Geometry check sheet. Reference: the model listing, model coordinates, mm. Face numbers are marked on the shaded views. A direction names the side the tool comes from. Round coordinates to 2 decimals unless told otherwise and drop trailing zeros. Write each loop counter-clockwise with the first axis right and the second up, starting at its lowest first coordinate (ties: lowest second). Pieces come first, ordered by that corner, then holes.
Item 1: Cross-section at D-D (z = 15). Enter the section's corners in (x, y) (3 decimals).
Item 2: Draft check along Z on the marked faces 1, 2 and 3. Enter one of: pulls with the +Z half, pulls with the -Z half, needs draft (parallel to the pull), parting line crosses it, or undercut.
Item 3: Scan lines: probe 1 along Y at (x, z) = (-0.2, -6.5); probe 2 along X at (y, z) = (5.75, 9) (3 decimals); probe 3 along Y at (x, z) = (-3, 14). Record each from-to range of solid material in increasing order.
Item 4: Access from +Z, -Z, +X, -X, +Y, -Y to the whole of each face (thin tool, end or side, straight path). Record for the marked faces 4, 5, 6, 7 and 8.
Item 5: Cross-section at C-C (y = 5.5). State how many separate pieces and enclosed holes the cut face has, then the cut area to 3 significant figures.
Item 6: Depth check by flat-ended pin: P1, Ø10, axis at x = -5.5, y = 4, coming from the -Z side; P2, Ø7, axis at y = 5, z = -6.5, coming from the +X side; P3, Ø3, axis at y = 6.5, z = -2.5, coming from the -X side; P4, Ø5, axis at y = 5.5, z = -2, coming from the +X side. Enter the tip coordinate at first touch or a pass-through.
Item 7: Cross-section at B-B (z = 10). Enter the section's corners in (x, y) (3 decimals), then the cut area to 3 significant figures.
Item 8: Cross-section at A-A (z = -4). Enter the section's corners in (x, y).
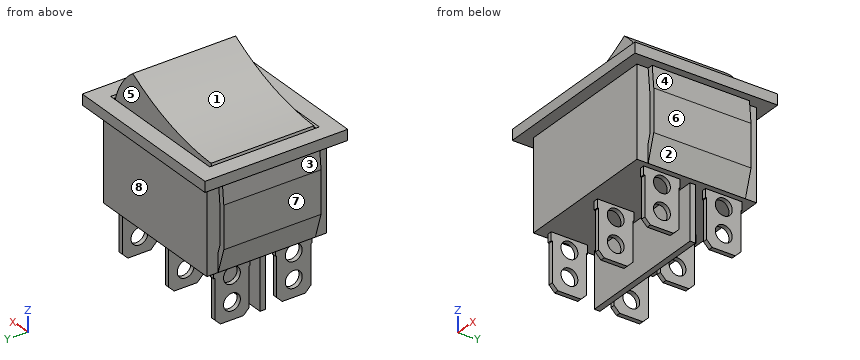
from build123d import *

# Parameters (mm, degrees)
SKETCH1_W                = 25.75
SKETCH1_H                = 21.3
BOSS_EXTRUDE1_DEPTH      = 16
SKETCH3_W                = 30.5
SKETCH3_H                = 25.4
BOSS_EXTRUDE3_DEPTH      = 1.87
SKETCH4_W                = 23.8
SKETCH4_H                = 1
BOSS_EXTRUDE4_DEPTH      = 9.8
SKETCH5_W                = 0.8
SKETCH5_H                = 6.5
BOSS_EXTRUDE5_DEPTH      = 9.5
SKETCH6_W                = 8
SKETCH6_H                = 0.2
CUT_EXTRUDE1_DEPTH       = 35.896266276
CHAMFER1_SIZE            = 1
SKETCH7_R                = 1.5
CUT_EXTRUDE2_DEPTH       = 35.896266276
CHAMFER1_OF_MIRROR1_SIZE = 1
BOSS_EXTRUDE6_START      = -2
BOSS_EXTRUDE6_DEPTH      = 17.3
SKETCH9_W                = 24
SKETCH9_H                = 18.9
CUT_EXTRUDE3_DEPTH       = 5
SKETCH10_R               = 12.5
BOSS_EXTRUDE7_DEPTH      = 9.15
CUT_EXTRUDE4_DEPTH       = 34.003475575
CUT_EXTRUDE4_DEPTH_BACK  = 34.003475575
SKETCH11_R               = 40
CHAMFER2_SIZE            = 0.3


with BuildPart() as part:
    # Sketch1 → Boss-Extrude1 (new body)
    with BuildSketch(Plane.XY):
        Rectangle(SKETCH1_W, SKETCH1_H)
    extrude(amount=BOSS_EXTRUDE1_DEPTH)

    # Sketch3 → Boss-Extrude3 (add)
    with BuildSketch(Plane.XY.offset(16)):
        Rectangle(SKETCH3_W, SKETCH3_H)
    extrude(amount=BOSS_EXTRUDE3_DEPTH)

    # Sketch4 → Boss-Extrude4 (add)
    with BuildSketch(Plane(origin=(0, 0, 0), x_dir=(-1, 0, 0), z_dir=(0, 0, -1))):
        Rectangle(SKETCH4_W, SKETCH4_H)
    extrude(amount=BOSS_EXTRUDE4_DEPTH)

    # Sketch5 → Boss-Extrude5 (add)
    with BuildSketch(Plane(origin=(0, 0, 0), x_dir=(-1, 0, 0), z_dir=(0, 0, -1))):
        with Locations((11.5, -5.5)):
            Rectangle(SKETCH5_W, SKETCH5_H)
        with Locations((0, -5.5)):
            Rectangle(SKETCH5_W, SKETCH5_H)
        with Locations((-11.5, -5.5)):
            Rectangle(SKETCH5_W, SKETCH5_H)
    boss_extrude5 = extrude(amount=BOSS_EXTRUDE5_DEPTH)

    # Sketch6 → Cut-Extrude1 (cut, through all)
    with BuildSketch(Plane(origin=(11.9, 0, 0), x_dir=(0, 0, -1), z_dir=(1, 0, 0))):
        with Locations((5.5, -2.35)):
            Rectangle(SKETCH6_W, SKETCH6_H)
        with Locations((5.5, -8.65)):
            Rectangle(SKETCH6_W, SKETCH6_H)
    cut_extrude1 = extrude(amount=-CUT_EXTRUDE1_DEPTH, mode=Mode.SUBTRACT)

    # Chamfer1
    chamfer1_edges = [part.edges().sort_by_distance(p)[0] for p in [
        (-11.5, -2.45, -9.5),
        (0, -2.45, -9.5),
        (-11.5, -8.55, -9.5),
        (0, -8.55, -9.5),
        (11.5, -8.55, -9.5),
        (11.5, -2.45, -9.5),
    ]]
    chamfer(chamfer1_edges, length=CHAMFER1_SIZE)

    # Sketch7 → Cut-Extrude2 (cut, through all)
    with BuildSketch(Plane(origin=(11.9, 0, 0), x_dir=(0, 0, -1), z_dir=(1, 0, 0))):
        with Locations((6.5, -5.5)):
            Circle(SKETCH7_R)
        with Locations((2, -5.5)):
            Circle(SKETCH7_R)
    cut_extrude2 = extrude(amount=-CUT_EXTRUDE2_DEPTH, mode=Mode.SUBTRACT)

    # Mirror1: Boss-Extrude5, Cut-Extrude1, Cut-Extrude2 across plane
    add(boss_extrude5.mirror(Plane(origin=(0, 0, 0), x_dir=(0, 0, 1), z_dir=(0, -1, 0))))
    add(cut_extrude1.mirror(Plane(origin=(0, 0, 0), x_dir=(0, 0, 1), z_dir=(0, -1, 0))), mode=Mode.SUBTRACT)
    add(cut_extrude2.mirror(Plane(origin=(0, 0, 0), x_dir=(0, 0, 1), z_dir=(0, -1, 0))), mode=Mode.SUBTRACT)

    # Chamfer1 of Mirror1
    chamfer1_of_mirror1_edges = [part.edges().sort_by_distance(p)[0] for p in [
        (-11.5, 2.45, -9.5),
        (0, 2.45, -9.5),
        (-11.5, 8.55, -9.5),
        (0, 8.55, -9.5),
        (11.5, 8.55, -9.5),
        (11.5, 2.45, -9.5),
    ]]
    chamfer(chamfer1_of_mirror1_edges, length=CHAMFER1_OF_MIRROR1_SIZE)

    # Sketch8 → Boss-Extrude6 (add)
    with BuildSketch(Plane(origin=(0, 10.65, 0), x_dir=(1, 0, 0), z_dir=(0, 1, 0)).offset(BOSS_EXTRUDE6_START)):
        Polygon((-12.875, 0), (-14.275, -4.5), (-14.275, -12), (-13.879867215, -16), (-12.875, -16), (-13.275, -11.95072831), (-13.275, -4.651963334), (-12.875, -3.366249048), align=None)
    boss_extrude6 = extrude(amount=-BOSS_EXTRUDE6_DEPTH)

    # Mirror2: Boss-Extrude6 across plane
    add(boss_extrude6.mirror(Plane.ZY))

    # Sketch9 → Cut-Extrude3 (cut)
    with BuildSketch(Plane.XY.offset(17.87)):
        Rectangle(SKETCH9_W, SKETCH9_H)
    extrude(amount=-CUT_EXTRUDE3_DEPTH, mode=Mode.SUBTRACT)

    # Sketch10 → Boss-Extrude7 (add, symmetric)
    with BuildSketch(Plane(origin=(0, 0, 0), x_dir=(-1, 0, 0), z_dir=(0, -1, 0))):
        with Locations((0, -13.87)):
            Circle(SKETCH10_R)
    extrude(amount=BOSS_EXTRUDE7_DEPTH, both=True)

    # Sketch11 → Cut-Extrude4 (cut, two sides: drawn at the far end of the back side and taken through both)
    with BuildSketch(Plane(origin=(0, 0, 0), x_dir=(-1, 0, 0), z_dir=(0, -1, 0)).offset(-CUT_EXTRUDE4_DEPTH_BACK)):
        with Locations((13, -58)):
            Circle(SKETCH11_R)
    extrude(amount=CUT_EXTRUDE4_DEPTH + CUT_EXTRUDE4_DEPTH_BACK, mode=Mode.SUBTRACT)

    # Chamfer2
    chamfer2_edges = [part.edges().sort_by_distance(p)[0] for p in [
        (-12, 0, 17.87),
        (0, 9.45, 17.87),
        (0, -9.45, 17.87),
        (12, 0, 17.87),
    ]]
    chamfer(chamfer2_edges, length=CHAMFER2_SIZE)


solid = part.part
Resolved:
1. outline: (-13.979, -8.65) - (-12.974, -8.65) - (-12.974, 8.65) - (-13.979, 8.65) - close; (-12.875, -10.65) - (12.875, -10.65) - (12.875, 10.65) - (-12.875, 10.65) - close; (12.974, -8.65) - (13.979, -8.65) - (13.979, 8.65) - (12.974, 8.65) - close; hole (-12, -9.45) - (12, -9.45) - (12, -9.15) - (-12, -9.15) - close; hole (-12, 9.15) - (12, 9.15) - (12, 9.45) - (-12, 9.45) - close
2. face 1: pulls with the +Z half
2. face 2: pulls with the -Z half
2. face 3: undercut
3. probe 1: y = -8.55 to -7, -4 to -2.45, -0.5 to 0.5, 2.45 to 4, 7 to 8.55
3. probe 2: x = -14.275 to -13.275, -12.875 to 12.875, 13.275 to 14.275
3. probe 3: y = -10.65 to -9.45, -9.15 to 9.15, 9.45 to 10.65
4. face 4: +X, +Y, -Y
4. face 5: +Z
4. face 6: -Z, +X, +Y, -Y
4. face 7: -Z, -X, +Y, -Y
4. face 8: -Z, +X, -X, +Y
5. separate pieces: 7
5. enclosed holes: 2
5. area: 562 mm2
6. P1: stops at z = -9.8
6. P2: stops at x = 11.9
6. P3: stops at x = -11.9
6. P4: stops at x = 13.03
7. outline: (-14.275, -8.65) - (-13.275, -8.65) - (-13.275, 8.65) - (-14.275, 8.65) - close; (-12.875, -10.65) - (12.875, -10.65) - (12.875, 10.65) - (-12.875, 10.65) - close; (13.275, -8.65) - (14.275, -8.65) - (14.275, 8.65) - (13.275, 8.65) - close
7. area: 583 mm2
8. outline: (-11.9, -8.55) - (-11.1, -8.55) - (-11.1, -2.45) - (-11.9, -2.45) - close; (-11.9, -0.5) - (11.9, -0.5) - (11.9, 0.5) - (-11.9, 0.5) - close; (-11.9, 2.45) - (-11.1, 2.45) - (-11.1, 8.55) - (-11.9, 8.55) - close; (-0.4, -8.55) - (0.4, -8.55) - (0.4, -2.45) - (-0.4, -2.45) - close; (-0.4, 2.45) - (0.4, 2.45) - (0.4, 8.55) - (-0.4, 8.55) - close; (11.1, -8.55) - (11.9, -8.55) - (11.9, -2.45) - (11.1, -2.45) - close; (11.1, 2.45) - (11.9, 2.45) - (11.9, 8.55) - (11.1, 8.55) - close
